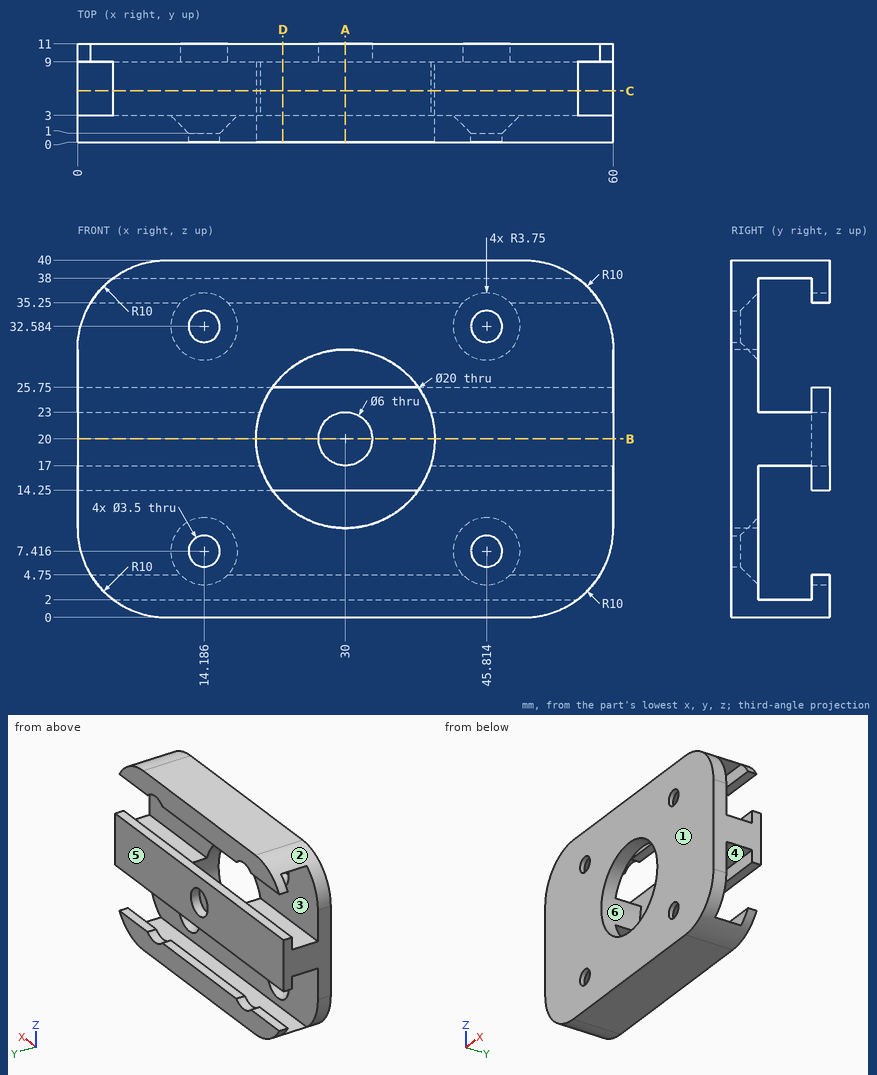
Source: three-view drawing plus pictorial views. Frame: mm from the lowest corner of the part. A direction names the side the tool comes from. Round coordinates to 2 decimals unless told otherwise and drop trailing zeros. Write each loop counter-clockwise with the first axis right and the second up, starting at its lowest first coordinate (ties: lowest second). Pieces come first, ordered by that corner, then holes. Notation, with made-up numbers: M -26.75,-37 L 28.25,-37 A17 ccw 28.25,-21 Z; hole C 38,-14.75 d11. An arc over 180 degrees is marked long. One line per item, written item: value. Start each with the question number.
Item 1: Section query C-C (y = 5.75). Return the cut outline in (x, z).
Item 2: Section query B-B (z = 20). Return the cut outline in (x, y), plus the area to 3 significant figures.
Item 3: Section query A-A (x = 30). Return the cut outline in (y, z), plus the area to 3 significant figures.
Item 4: Set-up query: the marked faces 4, 5 and 6. Return all of +Z, -Z, +X, -X, +Y, -Y with unobstructed straight access to the full face (end or side cutting, diameter ignored); none if empty.
Item 5: Pin query (flat end, axial travel): pin 1 (1.6 mm diameter, centred on x = 7, y = 9.5, fed in from -Z) (3 decimals); pin 2 (2 mm diameter, centred on x = 54, y = 10, fed in from -Z); pin 3 (5.5 mm diameter, centred on x = 45.81, z = 32.58, fed in from +Y) (1 decimal). Return the tip coordinate at first contact, or that it passes through.
Item 6: Mould query, pull axis Z, two halves, no side actions, for the marked faces 1, 2 and 3. Classes: pulls with the +Z half, pulls with the -Z half, needs draft (parallel to the pull), parting line crosses it, or undercut.
Item 7: Section query D-D (x = 23). Return the cut outline in (y, z).
Item 8: Ray query, L1, parallel to Z at x = 41, y = 9.5; L2, parallel to X at y = 10.05, z = 20; L3, parallel to Z at x = 15, y = 7.75. Return the intervals inside material, ascending. Write a range as from..to.
Result set:
1. outline: M 0,17 L 20.46,17 A10 cw 20.46,23 L 0,23 Z; M 4,2 A10 ccw 10,0 L 50,0 A10 ccw 56,2 Z; M 4,38 L 56,38 A10 ccw 50,40 L 10,40 A10 ccw Z; M 39.54,17 L 60,17 L 60,23 L 39.54,23 A10 cw Z
2. outline: M 0,0 L 20,0 L 20,9 L 27,9 L 27,11 L 0,11 Z; M 33,9 L 40,9 L 40,0 L 60,0 L 60,11 L 33,11 Z
2. area: 468 mm²
3. outline: M 0,0 L 11,0 L 11,4.75 L 9,4.75 L 9,2 L 3,2 L 3,10 L 0,10 Z; M 0,30 L 3,30 L 3,38 L 9,38 L 9,35.25 L 11,35.25 L 11,40 L 0,40 Z; M 9,14.25 L 11,14.25 L 11,17 L 9,17 Z; M 9,23 L 11,23 L 11,25.75 L 9,25.75 Z
3. area: 114 mm²
4. face 4: +X, -X
4. face 5: +Z, -Z, +X, -X, +Y
4. face 6: -Y
5. pin 1: stops at z = 0.245
5. pin 2: stops at z = 0.46
5. pin 3: stops at y = 2
6. face 1: needs draft
6. face 2: pulls with the +Z half
6. face 3: undercut
7. outline: M 0,0 L 11,0 L 11,4.75 L 9,4.75 L 9,2 L 3,2 L 3,12.86 L 0,12.86 Z; M 0,27.14 L 3,27.14 L 3,38 L 9,38 L 9,35.25 L 11,35.25 L 11,40 L 0,40 Z; M 9,14.25 L 11,14.25 L 11,25.75 L 9,25.75 Z
8. L1: z = 0..4.75, 14.25..25.75, 35.25..40
8. L2: x = 0..27, 33..60
8. L3: z = 0..2, 17..23, 38..40
